from build123d import *

# Parameters (mm, degrees)
SKETCH1_W           = 118
SKETCH1_H           = 80
BOSS_EXTRUDE1_DEPTH = 2.7
SKETCH3_W           = 5.5
SKETCH3_H           = 60
CUT_EXTRUDE1_DEPTH  = 2.7
SKETCH4_W           = 10
SKETCH4_H           = 60
CUT_EXTRUDE2_DEPTH  = 2.7
SKETCH7_W           = 4
SKETCH7_H           = 8
BOSS_EXTRUDE5_DEPTH = 8
SKETCH8_R           = 1.75
CUT_EXTRUDE4_DEPTH  = 131
FILLET1_R           = 3
SKETCH9_W           = 65.533885403
SKETCH9_H           = 5
CUT_EXTRUDE5_DEPTH  = 53
SKETCH10_R          = 1.75
CUT_EXTRUDE6_DEPTH  = 10


with BuildPart() as part:
    # Sketch1 → Boss-Extrude1 (new body)
    with BuildSketch(Plane.XY):
        with Locations((-14.766233766, 16)):
            Rectangle(SKETCH1_W, SKETCH1_H)
    extrude(amount=BOSS_EXTRUDE1_DEPTH)

    # Sketch3 → Cut-Extrude1 (cut)
    with BuildSketch(Plane.XY.offset(2.7)):
        with Locations((-71.016233766, 6)):
            Rectangle(SKETCH3_W, SKETCH3_H)
        with Locations((41.483766234, 6)):
            Rectangle(SKETCH3_W, SKETCH3_H)
    extrude(amount=-CUT_EXTRUDE1_DEPTH, mode=Mode.SUBTRACT)

    # Sketch4 → Cut-Extrude2 (cut)
    with BuildSketch(Plane.XY.offset(2.7)):
        with Locations((-63.266233766, 6)):
            Rectangle(SKETCH4_W, SKETCH4_H)
        with Locations((33.733766234, 6)):
            Rectangle(SKETCH4_W, SKETCH4_H)
    extrude(amount=-CUT_EXTRUDE2_DEPTH, mode=Mode.SUBTRACT)

    # Sketch7 → Boss-Extrude5 (add)
    with BuildSketch(Plane(origin=(0, 0, 0), x_dir=(-1, 0, 0), z_dir=(0, 0, -1))):
        with Locations((65.766233766, 44)):
            Rectangle(SKETCH7_W, SKETCH7_H)
        with Locations((-36.233766234, 44)):
            Rectangle(SKETCH7_W, SKETCH7_H)
    extrude(amount=BOSS_EXTRUDE5_DEPTH)

    # Sketch8 → Cut-Extrude4 (cut)
    with BuildSketch(Plane(origin=(38.233766234, 0, 0), x_dir=(0, 0, -1), z_dir=(1, 0, 0))):
        with Locations((4, 44)):
            Circle(SKETCH8_R)
    extrude(amount=-CUT_EXTRUDE4_DEPTH, mode=Mode.SUBTRACT)

    # Fillet1
    fillet1_edges = [part.edges().sort_by_distance(p)[0] for p in [
        (-65.766233766, 48, 0),
        (-65.766233766, 40, 0),
        (-65.766233766, 48, -8),
        (-65.766233766, 40, -8),
        (36.233766234, 40, 0),
        (36.233766234, 48, 0),
        (36.233766234, 40, -8),
        (36.233766234, 48, -8),
    ]]
    fillet(fillet1_edges, radius=FILLET1_R)

    # Sketch9 → Cut-Extrude5 (cut)
    with BuildSketch(Plane.XY.offset(2.7)):
        with Locations((-14.306023896, 53.5)):
            Rectangle(SKETCH9_W, SKETCH9_H)
    extrude(amount=-CUT_EXTRUDE5_DEPTH, mode=Mode.SUBTRACT)

    # Sketch10 → Cut-Extrude6 (cut)
    with BuildSketch(Plane(origin=(0, 0, 0), x_dir=(-1, 0, 0), z_dir=(0, 0, -1))):
        with Locations((9.766233766, -12.75)):
            Circle(SKETCH10_R)
        with Locations((10.266233766, 32.25)):
            Circle(SKETCH10_R)
        with Locations((-18.233766234, 38.25)):
            Circle(SKETCH10_R)
    extrude(amount=-CUT_EXTRUDE6_DEPTH, mode=Mode.SUBTRACT)


solid = part.part
Model file for the job. Use its own axes, mm. A direction names the side the tool comes from. Give positions to 0.01 mm unless a question says otherwise; leave off trailing zeros. Write each loop counter-clockwise with the first axis right and the second up, starting at its lowest first coordinate (ties: lowest second). Pieces come first, ordered by that corner, then holes. Notation, with made-up numbers: (65, -32) - (81, -32) arc R33 ccw to (81, 1) - close; hole circle Ø10 at (26.25, 1.5). An arc over 180 degrees is marked (long way). Answer as CSV lines item,"result".
1. Drill centre lines: L1, parallel to Z at x = -32, y = 28; L2, parallel to Y at x = 35.55, z = -4; L3, parallel to Y at x = -42, z = 1. Where is each one in solid material? Low to high. Write a range as [from, to].
Responses:
L1,"z = [0, 2.7]"
L2,"y = [40, 42.25], [45.75, 48]"
L3,"y = [-24, 51]"
2. Two-plate mould, pull along Y, no slides. Class faces 4 (the face through (36.21, 40.86, -7.1)), 5 (the face through (-58.266, 6, 1)), 6 (the face through (-11.935, 32.776, 1.331)): +Y half, -Y half, draft (parallel to the pull), parting line (faces both ways), or undercut.
Responses:
face 4,"-Y half"
face 5,"draft"
face 6,"undercut"
3. Band-saw the part on B-B (z = 1.5). Write the cut outline in (x, y).
Responses:
outline,"(-73.77, 36) - (-58.27, 36) - (-58.27, -24) - (28.73, -24) - (28.73, 36) - (44.23, 36) - (44.23, 56) - (18.46, 56) - (18.46, 51) - (-47.07, 51) - (-47.07, 56) - (-73.77, 56) - close; hole circle Ø3.5 at (-10.27, 32.25); hole circle Ø3.5 at (-9.77, -12.75); hole circle Ø3.5 at (18.23, 38.25)"
4. 3-axis set-ups, long thin cutter, end or side, ignore diameter. For faces 1 (the face through (18.461, 53, 1)), 2 (the face through (36, 36, 1)), 3 (the face through (-66, 36, 1)): which of +Z, -Z, +X, -X, +Y, -Y reach the whole face in a straight line?
Responses:
face 1,"+Z, -Z, +Y"
face 2,"+Z, -Z, +X, -Y"
face 3,"+Z, -Z, -X, -Y"
5. Band-saw the part on D-D (y = 38.25). Write the cut outline in (x, z).
Responses:
outline,"(-73.77, 0) - (-67.77, 0) - (-67.77, -0.27) - (-63.77, -0.27) - (-63.77, 0) - (16.48, 0) - (16.48, 2.7) - (-73.77, 2.7) - close; (19.98, 0) - (34.23, 0) - (34.23, -0.27) - (38.23, -0.27) - (38.23, 0) - (44.23, 0) - (44.23, 2.7) - (19.98, 2.7) - close"
6. Band-saw the part on C-C (x = -65.5). Write the cut outline in (y, z).
Responses:
outline,"(36, 0) - (37, 0) arc R3 cw to (40, -3) - (40, -5) arc R3 ccw to (43, -8) - (45, -8) arc R3 ccw to (48, -5) - (48, -3) arc R3 cw to (51, 0) - (56, 0) - (56, 2.7) - (36, 2.7) - close; hole circle Ø3.5 at (44, -4)"
7. Band-saw the part on A-A (y = -12.75). Write the cut outline in (x, z), and give its area (3 significant figures).
Responses:
outline,"(-58.27, 0) - (-11.52, 0) - (-11.52, 2.7) - (-58.27, 2.7) - close; (-8.02, 0) - (28.73, 0) - (28.73, 2.7) - (-8.02, 2.7) - close"
area,"225 mm2"
8. Pin check, flat tips, straight feed: pin 1 (3 mm diameter, centred on x = -2.5, z = 2, fed in from +Y); pin 2 (4 mm diameter, centred on y = 44, z = -3.5, fed in from +X); pin 3 (0.6 mm diameter, centred on x = -66, z = -4, fed in from -Y). Stop position of each tip, or through.
Responses:
pin 1,"stops at y = 51"
pin 2,"stops at x = 38.23"
pin 3,"stops at y = 40"
